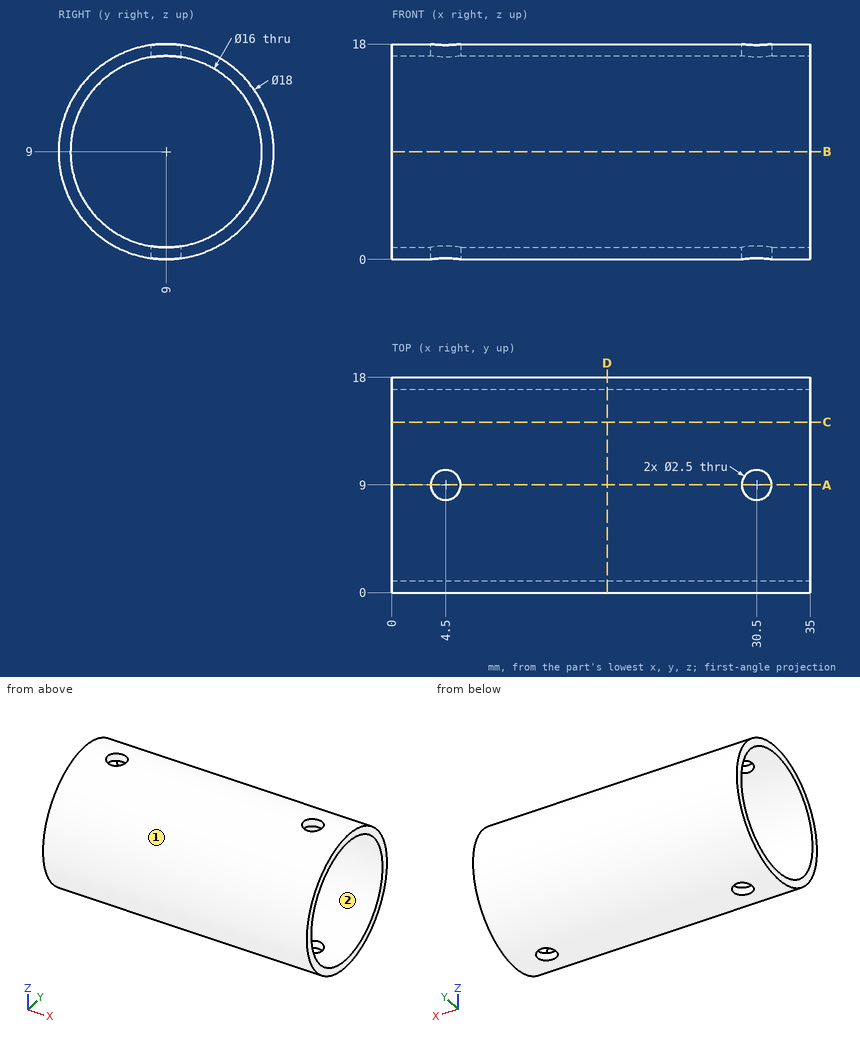
Answer from the drawing. Dimensions are ordinates in mm from the lowest x, y and z of the part. Give positions to 0.01 mm unless a question says otherwise; leave off trailing zeros. Write each loop counter-clockwise with the first axis right and the second up, starting at its lowest first coordinate (ties: lowest second). Pieces come first, ordered by that corner, then holes. Notation, with made-up numbers: (-36.5, 66.25) -> (-27.5, 66.25) arc R14 ccw to (-27.5, 78.25) -> close; hole circle Ø10 at (-15, -18). An arc over 180 degrees is marked (long way). Use a Markdown table: item, result.
(1) Flat-ended cylindrical pins translate along their axes: P1, Ø6, axis at x = 21.5, z = 6, coming from the -Y side; P2, Ø1, axis at x = 8.5, y = 2.5, coming from the -Z side; P3, Ø4, axis at x = 22.5, z = 13.5, coming from the -Y side; P4, Ø6, axis at x = 26.5, y = 12.5, coming from the +Z side. Find the tip coordinate at first contact, or state that the pin passes through.
Return value:
| item | result |
|---|---|
| P1 | y = 0 |
| P2 | z = 2.29 |
| P3 | y = 0.35 |
| P4 | z = 17.99 |
(2) Section A-A, the plane y = 9 is taken. Determine the outline of the cut face in (x, z).
Return value:
| item | result |
|---|---|
| outline | (0, 0) -> (3.25, 0) -> (3.25, 1) -> (0, 1) -> close; (0, 17) -> (3.25, 17) -> (3.25, 18) -> (0, 18) -> close; (5.75, 0) -> (29.25, 0) -> (29.25, 1) -> (5.75, 1) -> close; (5.75, 17) -> (29.25, 17) -> (29.25, 18) -> (5.75, 18) -> close; (31.75, 0) -> (35, 0) -> (35, 1) -> (31.75, 1) -> close; (31.75, 17) -> (35, 17) -> (35, 18) -> (31.75, 18) -> close |
(3) Section C-C, the plane y = 14.25 is taken. Determine the outline of the cut face in (x, z), then the cut area to 3 significant figures.
Return value:
| item | result |
|---|---|
| outline | (0, 1.69) -> (35, 1.69) -> (35, 2.96) -> (0, 2.96) -> close; (0, 15.04) -> (35, 15.04) -> (35, 16.31) -> (0, 16.31) -> close |
| area | 89.2 mm2 |
(4) Find the intervals of material crossed by probe 1 along Z at (x, y) = (26, 9.25); probe 2 along Z at (x, y) = (25, 3); probe 3 along Y at (x, z) = (2.5, 8.5), in increasing order. Write a range as from..to.
Return value:
| item | result |
|---|---|
| probe 1 | 0..1, 17..18 |
| probe 2 | 2.29..3.71, 14.29..15.71 |
| probe 3 | 0.01..1.02, 16.98..17.99 |
(5) Determine the mould class of the marked faces 1 and 2 for opening direction Z: released by +Z, released by -Z, zero draft, split by the parting line, or undercut.
Return value:
| item | result |
|---|---|
| face 1 | split by the parting line |
| face 2 | undercut |
(6) Section B-B, the plane z = 9 is taken. Determine the outline of the cut face in (x, y), then the cut area to 3 significant figures.
Return value:
| item | result |
|---|---|
| outline | (0, 0) -> (35, 0) -> (35, 1) -> (0, 1) -> close; (0, 17) -> (35, 17) -> (35, 18) -> (0, 18) -> close |
| area | 70.0 mm2 |
(7) Section D-D, the plane x = 18 is taken. Determine the outline of the cut face in (y, z).
Return value:
| item | result |
|---|---|
| outline | circle Ø18 at (9, 9); hole circle Ø16 at (9, 9) |
